```python
from build123d import *

# Parameters (mm, degrees)
F0_R     = 89.408
F0_R_2   = 9.525
F0_R_3   = 5.5
F1_DEPTH = 1.51892
F0_R_4   = 95
F2_DEPTH = 6.35


with BuildPart() as f1:
    # F0 (on Top) → F1 (new body)
    with BuildSketch(Plane.XY):
        Circle(F0_R)
        with Locations((-24.7515, -66.673965)):
            Circle(F0_R_2, mode=Mode.SUBTRACT)
        with Locations((-45.136415, -54.961427)):
            Circle(F0_R_2, mode=Mode.SUBTRACT)
        with Locations((-1.661818, -71.100582)):
            Circle(F0_R_2, mode=Mode.SUBTRACT)
        with Locations((-60.588964, -37.242876)):
            Circle(F0_R_2, mode=Mode.SUBTRACT)
        with Locations((-69.420541, -15.454541)):
            Circle(F0_R_2, mode=Mode.SUBTRACT)
        with Locations((-48.906072, -11.167962)):
            Circle(F0_R_2, mode=Mode.SUBTRACT)
        with Locations((-39.217583, -31.281119)):
            Circle(F0_R_2, mode=Mode.SUBTRACT)
        with Locations((-21.761934, -45.198954)):
            Circle(F0_R_2, mode=Mode.SUBTRACT)
        with Locations((-20.364587, -20.364587)):
            Circle(F0_R_2, mode=Mode.SUBTRACT)
        with Locations((21.609461, -67.75755)):
            Circle(F0_R_2, mode=Mode.SUBTRACT)
        with Locations((0.003733, -50.165)):
            Circle(F0_R_2, mode=Mode.SUBTRACT)
        with Locations((42.519327, -57.010186)):
            Circle(F0_R_2, mode=Mode.SUBTRACT)
        with Locations((21.768661, -45.195715)):
            Circle(F0_R_2, mode=Mode.SUBTRACT)
        with Locations((0, -28.799874)):
            Circle(F0_R_2, mode=Mode.SUBTRACT)
        with Locations((39.222239, -31.275281)):
            Circle(F0_R_2, mode=Mode.SUBTRACT)
        with Locations((20.364587, -20.364587)):
            Circle(F0_R_2, mode=Mode.SUBTRACT)
        with Locations((58.782813, -40.032927)):
            Circle(F0_R_2, mode=Mode.SUBTRACT)
        with Locations((68.622699, -18.680996)):
            Circle(F0_R_2, mode=Mode.SUBTRACT)
        with Locations((48.907733, -11.160683)):
            Circle(F0_R_2, mode=Mode.SUBTRACT)
        with Locations((-70.66606, 8.022618)):
            Circle(F0_R_2, mode=Mode.SUBTRACT)
        with Locations((-48.908564, 11.157043)):
            Circle(F0_R_2, mode=Mode.SUBTRACT)
        with Locations((-64.189413, 30.623091)):
            Circle(F0_R_2, mode=Mode.SUBTRACT)
        with Locations((-28.799874, 0)):
            Circle(F0_R_2, mode=Mode.SUBTRACT)
        with Locations((-20.364587, 20.364587)):
            Circle(F0_R_2, mode=Mode.SUBTRACT)
        with Locations((-39.224566, 31.272362)):
            Circle(F0_R_2, mode=Mode.SUBTRACT)
        with Locations((-21.772024, 45.194095)):
            Circle(F0_R_2, mode=Mode.SUBTRACT)
        with Locations((-50.698348, 49.877168)):
            Circle(F0_R_2, mode=Mode.SUBTRACT)
        with Locations((-31.667127, 63.680825)):
            Circle(F0_R_2, mode=Mode.SUBTRACT)
        with Locations((-9.175422, 70.525641)):
            Circle(F0_R_2, mode=Mode.SUBTRACT)
        Circle(F0_R_3, mode=Mode.SUBTRACT)
        with Locations((20.364587, 20.364587)):
            Circle(F0_R_2, mode=Mode.SUBTRACT)
        with Locations((28.799874, 0)):
            Circle(F0_R_2, mode=Mode.SUBTRACT)
        with Locations((0, 28.799874)):
            Circle(F0_R_2, mode=Mode.SUBTRACT)
        with Locations((21.765297, 45.197335)):
            Circle(F0_R_2, mode=Mode.SUBTRACT)
        with Locations((39.219911, 31.2782)):
            Circle(F0_R_2, mode=Mode.SUBTRACT)
        with Locations((48.906903, 11.164323)):
            Circle(F0_R_2, mode=Mode.SUBTRACT)
        with Locations((70.963711, 4.712336)):
            Circle(F0_R_2, mode=Mode.SUBTRACT)
        with Locations((65.550031, 27.590719)):
            Circle(F0_R_2, mode=Mode.SUBTRACT)
        with Locations((52.97325, 47.454074)):
            Circle(F0_R_2, mode=Mode.SUBTRACT)
        with Locations((0, 50.165)):
            Circle(F0_R_2, mode=Mode.SUBTRACT)
        with Locations((14.318945, 69.663636)):
            Circle(F0_R_2, mode=Mode.SUBTRACT)
        with Locations((34.607718, 62.131797)):
            Circle(F0_R_2, mode=Mode.SUBTRACT)
    extrude(amount=F1_DEPTH)

    # F0 (on Top) → F2 (join)
    with BuildSketch(Plane.XY):
        Circle(F0_R_4)
        Circle(F0_R, mode=Mode.SUBTRACT)
    extrude(amount=F2_DEPTH)


solid = f1.part
```
Check sheet for the modelled part. Datum: model origin and axes. Units: mm. A direction names the side the tool comes from. Round coordinates to 2 decimals unless told otherwise and drop trailing zeros. Order: outer loops, then holes, each group sorted by start corner. A loop starts at its lowest first (then second) coordinate and runs counter-clockwise, first axis right, second up. Notation, with made-up numbers: (-39.5, -13.5) - (-26.5, -13.5) arc R25 cw to (-26.5, 3.5) - close; hole circle Ø1 at (-8.5, 1). An arc over 180 degrees is marked (long way). Write item = value, one per line.
Q1. Tool access check on faces 1 (the face through (19, 1, 1.519)), 2 (the face through (80.05, 7.57, 0.75)). Record the directions out of +Z, -Z, +X, -X, +Y, -Y that give a thin tool (end or side, any length) a straight path to the whole face; none if there is none.
Computed:
face_1 = +Z
face_2 = +Z, -Z
Q2. Go/stop test with flat-tipped pins: pin 1 (3 mm diameter, centred on y = -39, z = 1.5, fed in from +X); pin 2 (25 mm diameter, centred on x = -48.91, y = 11.16, fed in from +Z); pin 3 (2 mm diameter, centred on x = -16.5, z = 1, fed in from -Y); pin 4 (17 mm diameter, centred on x = 0, y = 28.8, fed in from -Z). Record where each tip stops, or that it passes through.
Computed:
pin_1 = 87.29
pin_2 = 1.52
pin_3 = -93.73
pin_4 = through
Q3. Section check A-A (z = 4). Record the boundary of the cut face in (x, y).
Computed:
outline = circle Ø190 at (0, 0); hole circle Ø178.82 at (0, 0)
Q4. Thickness scan on line 1 along Y through (x, z) = (-74.5, 1.25); line 2 along Z through (x, y) = (68.5, 55); line 3 along Y through (x, z) = (-17, 6). Record the ranges inside material, lowest first.
Computed:
line_1 = -58.95 to -23.51, -7.4 to -0.7, 16.74 to 58.95
line_2 = 0 to 1.52
line_3 = -93.47 to -87.78, 87.78 to 93.47
Q5. Draft check along X on faces 3 (the face through (-23.837, 35.896, 0.749)), 4 (the face through (-20.59, -92.74, 3.13)), 5 (the face through (41, 1, 0)). Enter one of: pulls with the +X half, pulls with the -X half, needs draft (parallel to the pull), parting line crosses it, or undercut.
Computed:
face_3 = undercut
face_4 = parting line crosses it
face_5 = needs draft
